Input: part model. Units: mm. Frame: model coordinates. A direction names the side the tool comes from. Round coordinates to 2 decimals unless told otherwise and drop trailing zeros. Loops run counter-clockwise (first coordinate to the right, second up) from the corner with the lowest first, then second, coordinate; pieces in that order, holes last. Notation, with made-up numbers: (59.5, 83.5) -> (115.5, 83.5) arc R21 cw to (115.5, 103.5) -> close; hole circle Ø8 at (14.5, 55.5). An arc over 180 degrees is marked (long way). Answer in a Markdown table with one row per item. Add a question column.
Q1. Section A-A, the plane x = 0. Output: boundary loops of the cut face in (y, z) (3 decimals), and give its area (3 significant figures).
Q2. Reachability of faces 1 (the face through (-16, 27.53, 0)), 2 (the face through (22.35, 8, 0)) from +Z, -Z, +X, -X, +Y, -Y: full face, straight path, thin tool, end or side. Return the list, or none.
Q3. Section C-C, the plane z = 9. Output: boundary loops of the cut face in (x, y).
Q4. Section B-B, the plane y = 36.5. Output: boundary loops of the cut face in (x, z) (3 decimals).
Q5. Section D-D, the plane x = -7. Output: boundary loops of the cut face in (y, z), and give its area (3 significant figures).
Q6. Pin query (flat end, axial travel): pin 1 (12 mm diameter, centred on x = 14.5, y = 9.5, fed in from -Z); pin 2 (1.9 mm diameter, centred on x = -15.5, z = -0.5, fed in from +Y); pin 3 (1 mm diameter, centred on y = 16, z = -7, fed in from +X); pin 4 (10 mm diameter, centred on x = -5.5, z = -11, fed in from -Y). Return the tip coordinate at first contact, or that it passes through.
Q7. Ray query, L1, parallel to X at y = 30, z = 0; L2, parallel to X at y = 35.45, z = 0 (3 decimals); L3, parallel to Z at x = 0.5, y = 7.5. Return the intervals inside material, ascending. Write a range as from..to.
```python
from build123d import *

# Parameters (mm, degrees)
SKETCH2_R           = 19.1
BOSS_EXTRUDE1_DEPTH = 33.53
SKETCH3_R           = 11.955
SKETCH3_R_2         = 8.075
BOSS_EXTRUDE2_DEPTH = 1
SKETCH3_2_R         = 8.075
SKETCH3_2_R_2       = 4
BOSS_EXTRUDE3_DEPTH = 6
SKETCH4_R           = 1.2
CUT_EXTRUDE1_DEPTH  = 6
SKETCH5_R           = 8.24
BOSS_EXTRUDE4_DEPTH = 22.35
BOSS_EXTRUDE4_TAPER = 7
FILLET1_R           = 2.5


with BuildPart() as part:
    # Sketch2 → Boss-Extrude1 (new body)
    with BuildSketch(Plane(origin=(0, 0, 0), x_dir=(1, 0, 0), z_dir=(0, 1, 0))):
        with Locations(Location((0, 0, 0), (0, 0, 270))):
            Circle(SKETCH2_R)
    extrude(amount=BOSS_EXTRUDE1_DEPTH)

    # Sketch3 → Boss-Extrude2 (add)
    with BuildSketch(Plane(origin=(0, 33.53, 0), x_dir=(1, 0, 0), z_dir=(0, 1, 0))):
        with Locations(Location((0, 0, 0), (0, 0, 270))):
            Circle(SKETCH3_R)
        with Locations(Location((0, 0, 0), (0, 0, 270))):
            Circle(SKETCH3_R_2, mode=Mode.SUBTRACT)
    extrude(amount=BOSS_EXTRUDE2_DEPTH)

    # Sketch3_2 → Boss-Extrude3 (add)
    with BuildSketch(Plane(origin=(0, 33.53, 0), x_dir=(1, 0, 0), z_dir=(0, 1, 0))):
        with Locations(Location((0, 0, 0), (0, 0, 270))):
            Circle(SKETCH3_2_R)
        with Locations(Location((0, 0, 0), (0, 0, 270))):
            Circle(SKETCH3_2_R_2, mode=Mode.SUBTRACT)
    extrude(amount=BOSS_EXTRUDE3_DEPTH)

    # Sketch4 → Cut-Extrude1 (cut)
    with BuildSketch(Plane(origin=(0, 33.53, 0), x_dir=(1, 0, 0), z_dir=(0, 1, 0))):
        with Locations(Location((-15.5275, 0, 0), (0, 0, 270))):
            Circle(SKETCH4_R)
        with Locations(Location((15.5275, 0, 0), (0, 0, 270))):
            Circle(SKETCH4_R)
    extrude(amount=-CUT_EXTRUDE1_DEPTH, mode=Mode.SUBTRACT)

    # Sketch5 → Boss-Extrude4 (add)
    with BuildSketch(Plane(origin=(0, 0, 0), x_dir=(0, 0, -1), z_dir=(1, 0, 0))):
        with Locations((0, 8.24)):
            Circle(SKETCH5_R)
    extrude(amount=BOSS_EXTRUDE4_DEPTH, taper=BOSS_EXTRUDE4_TAPER)

    # Fillet1
    fillet1_edges = [part.edges().sort_by_distance(p)[0] for p in [
        (18.128459183, 8.262192057, 6.014064156),
    ]]
    fillet(fillet1_edges, radius=FILLET1_R - 0.0001)  # a hair under: the kernel refuses the full size


solid = part.part
```
Answer block:
| question | item | result |
|---|---|---|
| 1 | outline | (0, -19.1) -> (33.53, -19.1) -> (33.53, -11.955) -> (34.53, -11.955) -> (34.53, -8.075) -> (39.53, -8.075) -> (39.53, -4) -> (33.53, -4) -> (33.53, 4) -> (39.53, 4) -> (39.53, 8.075) -> (34.53, 8.075) -> (34.53, 11.955) -> (33.53, 11.955) -> (33.53, 19.1) -> (0, 19.1) -> close |
| 1 | area | 1,340 mm^2 |
| 2 | face 1 | +Y |
| 2 | face 2 | +Z, -Z, +X, +Y, -Y |
| 3 | outline | (-16.85, 0) -> (16.85, 0) -> (16.85, 33.53) -> (7.87, 33.53) -> (7.87, 34.53) -> (-7.87, 34.53) -> (-7.87, 33.53) -> (-16.85, 33.53) -> close |
| 4 | outline | circle Ø16.15 at (0, 0); hole circle Ø8 at (0, 0) |
| 5 | outline | (0, -17.77) -> (33.53, -17.77) -> (33.53, -9.69) -> (34.53, -9.69) -> (34.53, -4.03) -> (39.53, -4.03) -> (39.53, 4.03) -> (34.53, 4.03) -> (34.53, 9.69) -> (33.53, 9.69) -> (33.53, 17.77) -> (0, 17.77) -> close |
| 5 | area | 1,250 mm^2 |
| 6 | pin 1 | z = -17.1 |
| 6 | pin 2 | y = 33.53 |
| 6 | pin 3 | x = 17.96 |
| 6 | pin 4 | y = 0 |
| 7 | L1 | -19.1..-16.73, -14.33..14.33, 16.73..19.1 |
| 7 | L2 | -8.075..-4, 4..8.075 |
| 7 | L3 | -19.09..19.09 |
